Verification items for this drawing (mm, ordinates from the low corner). A direction names the side the tool comes from. Round coordinates to 2 decimals unless told otherwise and drop trailing zeros. Order: outer loops, then holes, each group sorted by start corner. A loop starts at its lowest first (then second) coordinate and runs counter-clockwise, first axis right, second up.
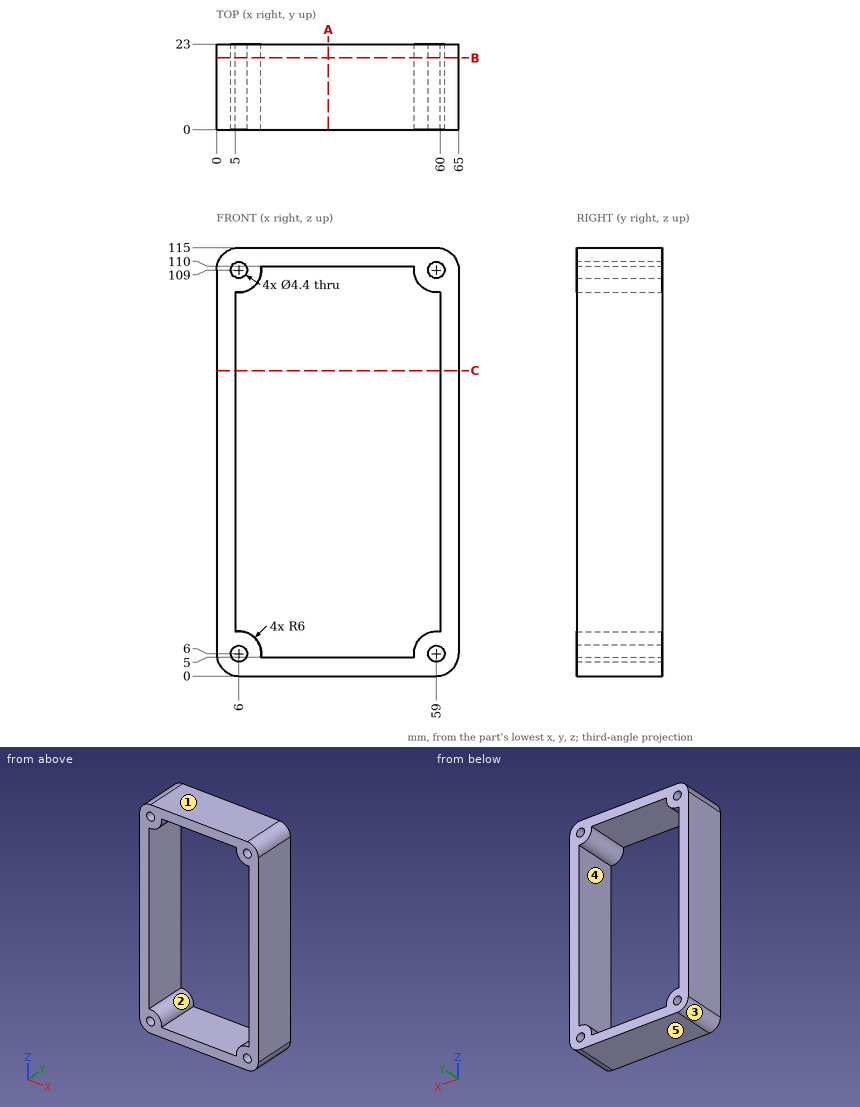
Item 1: Sectioned sample at A-A (x = 30). Record the cut outline in (y, z), and give its area (3 significant figures).
Answer:
outline: (0, 0) - (23, 0) - (23, 5) - (0, 5) - close; (0, 110) - (23, 110) - (23, 115) - (0, 115) - close
area: 230 mm2
Item 2: Scan lines: line 1 along X through (y, z) = (17, 6); line 2 along X through (y, z) = (21, 46.5); line 3 along Z through (x, y) = (20, 2). Record each from-to range of solid material in increasing order.
Answer:
line 1: x = 0 to 3.8, 8.2 to 12, 53 to 56.8, 61.2 to 65
line 2: x = 0 to 5, 60 to 65
line 3: z = 0 to 5, 110 to 115
Item 3: Go/stop test with a flat-tipped pin: P1, Ø4, axis at x = 6, z = 6, coming from the +Y side. Record where the tip stops, or that it passes through.
Answer:
P1: passes through
Item 4: Access from +Z, -Z, +X, -X, +Y, -Y to the whole of each face (thin tool, end or side, straight path). Record for the marked faces 4 and 5.
Answer:
face 4: +Y, -Y
face 5: -Z, +X, -X, +Y, -Y
Item 5: Sectioned sample at B-B (y = 19.25). Record the cut outline in (x, z).
Answer:
outline: (0, 6) arc R6 ccw to (6, 0) - (59, 0) arc R6 ccw to (65, 6) - (65, 109) arc R6 ccw to (59, 115) - (6, 115) arc R6 ccw to (0, 109) - close; hole circle Ø4.4 at (6, 6); hole circle Ø4.4 at (6, 109); hole (5, 11.92) arc R6 cw to (11.92, 5) - (53.08, 5) arc R6 cw to (60, 11.92) - (60, 103.08) arc R6 cw to (53.08, 110) - (11.92, 110) arc R6 cw to (5, 103.08) - close; hole circle Ø4.4 at (59, 6); hole circle Ø4.4 at (59, 109)
Item 6: Sectioned sample at C-C (z = 82). Record the cut outline in (x, y), and give its area (3 significant figures).
Answer:
outline: (0, 0) - (5, 0) - (5, 23) - (0, 23) - close; (60, 0) - (65, 0) - (65, 23) - (60, 23) - close
area: 230 mm2
Item 7: Release check for a two-part mould opening along Z. For the marked faces 1, 2 and 3 record: released by +Z, released by -Z, zero draft, split by the parting line, or undercut.
Answer:
face 1: released by +Z
face 2: undercut
face 3: released by -Z
